Part model, mm, in its own coordinate system. Face numbers are marked on the shaded views. A direction names the side the tool comes from. Coordinates: 2 decimals unless noted, no trailing zeros. Loops run counter-clockwise (first coordinate to the right, second up) from the corner with the lowest first, then second, coordinate; pieces in that order, holes last. Notation, with made-up numbers: (74.5, 72) - (127.5, 72) arc R10 ccw to (127.5, 88) - close; hole circle Ø1 at (-32.75, 27.5). An arc over 180 degrees is marked (long way). Use a Markdown table: item, result. Add a question column.
1) Pull direction X, two halves, no side cores. Call the marked faces 1, 2 and 3: +X half, -X half, draft (parallel to the pull), parting line (faces both ways), or undercut.
2) Band-saw the part on A-A (y = -78). Give the cut face in (x, z) (3 decimals).
3) Drop flat-ended pins along their axis: P1, Ø1.5, axis at x = -32.5, z = 13.5, coming from the +Y side; P2, Ø7, axis at y = 0.5, z = 6, coming from the +X side; P3, Ø2.5, axis at y = -16, z = 11, coming from the +X side; P4, Ø6.5, axis at x = -9.5, z = 4.5, coming from the -Y side. Give the stop position or say it passes through.
4) Tool access for the marked faces 4, 5 and 6: list every direction of +Z, -Z, +X, -X, +Y, -Y with a clear straight run to the whole face (end or side of a thin tool).
5) Band-saw the part on B-B (y = 0). Give the number of separate pieces and of enclosed holes in the cut face, plus the area to 3 significant figures.
6) Probe probe 1 along Z at (x, y) = (27, 0); probe 2 along Y at (x, z) = (0, 7.45); probe 3 along Y at (x, z) = (0, 1.75). List the from-to ranges inside material, lowest first. Write a range as [from, to].
7) Band-saw the part on C-C (x = -51.5). Give the cut face in (y, z).
Autodesk Inventor part; units mm, degrees
sketch "Boceto1" plane through (0, 0, 0) normal (0, 0, 1) x (1, 0, 0)
  line L0 (-37.2583, 0) -> (45.75, 0) construction
  line L1 (0, -58.9269) -> (0, 58.9269) construction
  line L2 (31.75, -21.0606) -> (31.75, 21.0606)
  line L3 (0, 38.1) -> (-25.4, 38.1)
  line L4 (0, -38.1) -> (-25.4, -38.1)
  arc A0 (31.75, 21.0606) -> (0, 38.1) centre (0, 0) ccw
  arc A1 (0, -38.1) -> (31.75, -21.0606) centre (0, 0) ccw
  line L5 (-25.4, 38.1) -> (-25.4, -38.1)
  dimension "d2" = 31.75
  dimension "d3" = 25.4
extrude "Cabezal" add sketch "Boceto1" along normal blind 9.652
sketch "Boceto3" plane through (0, 0, 9.652) normal (0, 0, 1) x (1, 0, 0)
  point P0 (0, 0)
  point P1 (0, 0)
hole "Broca y barreno" at (0, 0, 9.652) direction (0, 0, -1) diameter 15.875 end through all counterbore diameter 25.4 counterbore depth 3.048
sketch "Boceto4" plane through (0, 0, 0) normal (0, 0, 1) x (1, 0, 0)
  line L0 (-36.83, 0) -> (43.18, 0) construction
  line L1 (0, -53.34) -> (0, 53.34) construction
  line L2 (-12.7, 17.526) -> (-227.4102, 17.526) construction
  arc A0 (-119.126, 17.526) -> (-160.274, 17.526) centre (-139.7, 17.526) ccw
  line L3 (-12.7, 17.526) -> (-138.4236, -108.1976) construction
  line L4 (-12.7, 17.526) -> (165.1, 17.526) construction
  arc A1 (-117.0506, -86.8246) -> (-87.9545, -57.7285) centre (-102.5026, -72.2766) ccw
  arc A2 (-160.274, 17.526) -> (-117.0506, -86.8246) centre (-12.7, 17.526) ccw
  arc A3 (-119.126, 17.526) -> (-87.9545, -57.7285) centre (-12.7, 17.526) ccw
  line L5 (-25.4, 38.1) -> (-25.4, -38.1)
  point P0 (0, 0)
  dimension "d14" = 17.526
  dimension "d15" = 12.7
  dimension "d19" = 41.148
  dimension "d21" = 135
  dimension "d22" = 41.148
  dimension "d25" = 12.7
extrude "Mango" add sketch "Boceto4" along normal blind 15.875 and the other way blind 3.175
sketch "Boceto8" plane through (31.75, -21.0606, 0) normal (1, 0, 0) x (0, 0, -1)
  circle A0 centre (-4.826, 21.0606) radius 3.175
  line L0 (-9.652, 0) -> (-9.652, 42.1211) construction
  line L1 (0, 0) -> (-9.652, 0) construction
  line L2 (0, 42.1211) -> (-9.652, 42.1211) construction
  line L3 (-6.604, 33.7606) -> (-6.604, 8.3606)
  line L4 (-6.604, 28.9981) -> (-6.604, 13.1231)
  point P0 (0, 21.0606)
  dimension "d36" = 6.35
  dimension "d37" = 4.826
  dimension "d38" = 42.1211
  dimension "d39" = 21.0606
extrude "AgujeroLateral" cut sketch "Boceto8" against normal blind 9.652
sketch "Boceto9" plane through (0, 0, 0) normal (0, 0, 1) x (1, 0, 0)
  arc A0 (-160.274, 17.526) -> (-119.126, 17.526) centre (-139.7, 17.526) ccw
  line L0 (-25.4, 38.1) -> (-25.4, -38.1)
  line L1 (-139.7, 38.1) -> (-25.4, 38.1)
  arc A1 (-119.126, 17.526) -> (-160.274, 17.526) centre (-139.7, 17.526) ccw
  line L2 (-25.4, -38.1) -> (0, -38.1)
  line L3 (-25.4, 38.1) -> (-25.4, -38.1)
  line L4 (-25.4, -38.1) -> (-33.9695, -38.1)
  arc A2 (-87.9545, -57.7285) -> (-117.0506, -86.8246) centre (-102.5026, -72.2766) ccw
  arc A3 (-160.274, 17.526) -> (-117.0506, -86.8246) centre (-12.7, 17.526) ccw
  arc A4 (-117.0506, -86.8246) -> (-87.9545, -57.7285) centre (-102.5026, -72.2766) ccw
  arc A5 (-119.126, 17.526) -> (-87.9545, -57.7285) centre (-12.7, 17.526) ccw
  arc A6 (-119.126, 17.526) -> (-160.274, 17.526) centre (-139.7, 17.526) ccw
  line L5 (10.5292, 11.6592) -> (185.2985, 11.6592) construction
  arc A7 (-117.0506, -86.8246) -> (-87.9545, -57.7285) centre (-102.5026, -72.2766) ccw construction
  line L6 (-87.9545, -86.8246) -> (-42.9497, -41.8197)
  line L7 (-139.7, 17.526) -> (0, 17.526) construction
  line L8 (0, 17.526) -> (-119.126, -101.6) construction
  arc A8 (-33.9695, -38.1) -> (-42.9497, -41.8197) centre (-33.9695, -50.8) ccw
  line L9 (-25.4, 38.1) -> (-25.4, -38.1)
  arc A9 (-87.9545, -57.7285) -> (-119.126, 17.526) centre (-12.7, 17.526) ccw
  arc A10 (-119.126, 17.526) -> (-87.9545, -57.7285) centre (-12.7, 17.526) ccw
  circle A11 centre (-139.7, 17.526) radius 20.574
  circle A12 centre (-102.5026, -72.2766) radius 20.574
  point P0 (0, 0)
  point P1 (-87.9545, -57.7285)
  point P2 (-119.126, 17.526)
  dimension "d47" = 45
  dimension "d48" = 12.7
extrude "BloqueCentral" add sketch "Boceto9" along normal blind 12.7 contours A9 L1 L0 L4 A8 L6 A5 | A1 L1 A9 | A9 L6 A4
sketch "Boceto10" plane through (0, 0, 15.875) normal (0, 0, 1) x (1, 0, 0)
  arc A0 (-160.274, 17.526) -> (-117.0506, -86.8246) centre (-12.7, 17.526) ccw construction
  arc A1 (-117.0506, -86.8246) -> (-87.9545, -57.7285) centre (-102.5026, -72.2766) ccw construction
  arc A2 (-119.126, 17.526) -> (-87.9545, -57.7285) centre (-12.7, 17.526) ccw construction
  arc A3 (-119.126, 17.526) -> (-160.274, 17.526) centre (-139.7, 17.526) ccw construction
  arc A4 (-150.876, 17.526) -> (-110.4052, -80.1792) centre (-12.7, 17.526) ccw
  arc A5 (-110.4052, -80.1792) -> (-94.5999, -64.3739) centre (-102.5026, -72.2766) ccw
  arc A6 (-128.524, 17.526) -> (-94.5999, -64.3739) centre (-12.7, 17.526) ccw
  arc A7 (-128.524, 17.526) -> (-150.876, 17.526) centre (-139.7, 17.526) ccw
  point P0 (0, 0)
  dimension "d52" = 22.352
extrude "HuecoMango" cut sketch "Boceto10" against normal blind 22.352
sketch "Boceto11" plane through (0, 0, 12.7) normal (0, 0, 1) x (1, 0, 0)
  arc A0 (-105.5616, 17.526) -> (-118.1445, 3.1051) centre (-105.5616, 4.826) ccw
  arc A1 (-97.4576, -46.8374) -> (-78.3631, -48.1371) centre (-87.3433, -39.1568) ccw
  arc A2 (-56.0605, -25.8345) -> (-74.021, 17.526) centre (-74.021, -7.874) ccw
  arc A3 (-128.524, 17.526) -> (-150.876, 17.526) centre (-139.7, 17.526) ccw construction
  arc A4 (-128.524, 17.526) -> (-94.5999, -64.3739) centre (-12.7, 17.526) ccw construction
  arc A5 (-110.4052, -80.1792) -> (-94.5999, -64.3739) centre (-102.5026, -72.2766) ccw construction
  arc A6 (-150.876, 17.526) -> (-110.4052, -80.1792) centre (-12.7, 17.526) ccw construction
  arc A7 (-119.126, 17.526) -> (-160.274, 17.526) centre (-139.7, 17.526) ccw construction
  arc A8 (-160.274, 17.526) -> (-117.0506, -86.8246) centre (-12.7, 17.526) ccw construction
  arc A9 (-117.0506, -86.8246) -> (-87.9545, -57.7285) centre (-102.5026, -72.2766) ccw construction
  arc A10 (-119.126, 17.526) -> (-87.9545, -57.7285) centre (-12.7, 17.526) ccw construction
  line L0 (-139.7, 17.526) -> (-12.7, 17.526) construction
  line L1 (-12.7, 17.526) -> (-102.5026, -72.2766) construction
  arc A11 (-119.126, 17.526) -> (-87.9545, -57.7285) centre (-12.7, 17.526) ccw
  line L2 (-150.876, 17.526) -> (-150.876, 17.526)
  line L3 (-110.0905, -79.8645) -> (-110.4052, -80.1792)
  line L4 (-78.3631, -48.1371) -> (-56.0605, -25.8345)
  line L5 (-105.5616, 17.526) -> (-74.021, 17.526)
  arc A12 (-118.1445, 3.1051) -> (-97.4576, -46.8374) centre (-12.7, 17.526) ccw
  line L6 (-87.9545, -86.8246) -> (-42.9497, -41.8197)
  line L7 (-25.4, 38.1) -> (-139.7, 38.1)
  point P0 (0, 0)
  dimension "d57" = 25.4
  dimension "d58" = 25.4
  dimension "d59" = 50.8
  dimension "d60" = 20.574
  dimension "d61" = 20.574
extrude "HuecoCentral" cut sketch "Boceto11" against normal blind 12.7
equation "\"d39\" = 0.5 * d38"
properties part number "Pieza2A01209499"
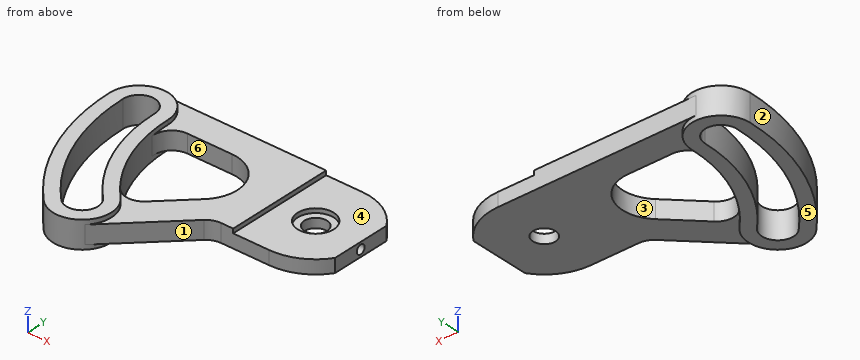
Answer block:
| question | item | result |
|---|---|---|
| 1 | face 1 | +X half |
| 1 | face 2 | -X half |
| 1 | face 3 | undercut |
| 2 | outline | (-125.185, -3.175) - (-112.537, -3.175) - (-112.537, 15.875) - (-125.185, 15.875) - close; (-92.903, -3.175) - (-82.741, -3.175) - (-82.741, 0) - (-79.13, 0) - (-79.13, 12.7) - (-82.741, 12.7) - (-82.741, 15.875) - (-92.903, 15.875) - close |
| 3 | P1 | through |
| 3 | P2 | x = 31.75 |
| 3 | P3 | x = -25.4 |
| 3 | P4 | y = -38.1 |
| 4 | face 4 | +Z, +X, +Y, -Y |
| 4 | face 5 | -Z, +X, -X, +Y, -Y |
| 4 | face 6 | +Z, -Z |
| 5 | separate pieces | 4 |
| 5 | enclosed holes | 0 |
| 5 | area | 981 mm2 |
| 6 | probe 1 | [0, 1.65], [8, 9.65] |
| 6 | probe 2 | [-38.1, -12.7], [12.7, 38.1] |
| 6 | probe 3 | [-38.1, -7.94], [7.94, 38.1] |
| 7 | outline | (-50.37, 0) - (-19.62, 0) - (-19.62, 12.7) - (-50.37, 12.7) - close; (3.87, 0) - (38.1, 0) - (38.1, 12.7) - (3.87, 12.7) - close |
